The figure shows three views and two pictorial views of one solid part (mm, origin at its lowest corner). Answer the questions. Coordinates: 2 decimals unless noted, no trailing zeros. Order: outer loops, then holes, each group sorted by start corner. A loop starts at its lowest first (then second) coordinate and runs counter-clockwise, first axis right, second up. Notation, with made-up numbers: (16.5, 75) -> (45.5, 75) arc R12 ccw to (45.5, 96) -> close; hole circle Ø8 at (79.25, 5). An arc over 180 degrees is marked (long way). Write item = value, one per line. Start each with the question number.
Q1. Straight lines are drawn through the part: L1, parallel to Z at x = 28.43, y = 0.5; L2, parallel to Z at x = 6, y = 0.55. For each, find the intervals that lie inside material, in ascending order. Write a range as from..to.
Q2. The part is cut by section A-A, the plane x = 5.57. Determine the outline of the cut face in (y, z).
Q3. The part is cut by section B-B, the plane z = 6.7. Count the separate pieces of the cut face and the enclosed holes in it, plus the area to 3 significant figures.
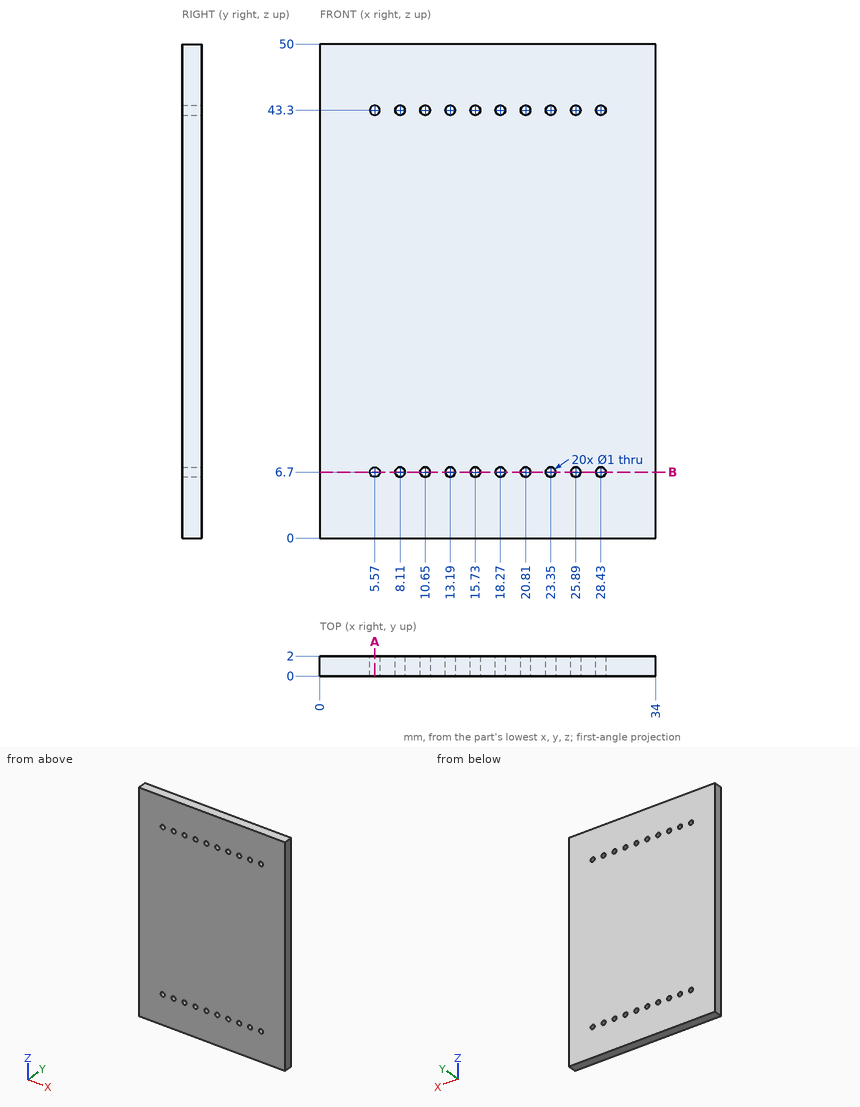
Model answer:
q1.L1 = 0..6.2, 7.2..42.8, 43.8..50
q1.L2 = 0..6.44, 6.96..43.04, 43.56..50
q2.outline = (0, 0) -> (2, 0) -> (2, 6.2) -> (0, 6.2) -> close; (0, 7.2) -> (2, 7.2) -> (2, 42.8) -> (0, 42.8) -> close; (0, 43.8) -> (2, 43.8) -> (2, 50) -> (0, 50) -> close
q3.separate_pieces = 11
q3.enclosed_holes = 0
q3.area = 48.0 mm2
